Can you work these out from the model? Positions are in its coordinate system, mm. A direction names the side the tool comes from. Coordinates: 2 decimals unless noted, no trailing zeros. Order: outer loops, then holes, each group sorted by start corner. A loop starts at its lowest first (then second) coordinate and runs counter-clockwise, first axis right, second up. Notation, with made-up numbers: (23, 10.25) - (69, 10.25) arc R23 ccw to (69, 31.25) - close; hole circle Ø3 at (58.5, -34). An arc over 180 degrees is marked (long way). Return JSON: item names as keys, results as strings. Group by question number.
1) Imagine slicing it at A-A (z = 50). Write out the boundary of the cut face in (x, y).
2) Which directions (+Z, -Z, +X, -X, +Y, -Y) give clear straight access to the entire face, cutting with the end or side of a thin tool? Please do faces 1 (the face through (-1, 35, 120)), 2 (the face through (43, 5, 54)).
3) If I drill on line 1 along Z through (x, y) = (-91, 3); line 2 along X through (y, z) = (6, -111); line 3 along X through (y, z) = (4, -50), over which ranges is the centre line in solid material (lowest first)?
4) Imagine slicing it at C-C (y = 46.5). Write out the boundary of the cut face in (x, z).
5) Imagine slicing it at B-B (x = -40). Write out the boundary of the cut face in (y, z), and give its area (3 significant figures).
6) For pin 1 Ø1.5 at (x, z) = (68.5, 76.5) entering from +Y; pin 2 Ø8 at (x, z) = (40, 50) entering from -Y, each with a flat end and sliding along its axis, tell me the tip position at first contact or that it passes through.
7) Imagine slicing it at D-D (x = 54.5). Write out the boundary of the cut face in (y, z).
8) If we mould it in two halves opening along X, with no side actions, what happens to faces 3 (the face through (-103, 30, 2)), 4 (the face through (103, 30, 2)), 5 (the face through (100, 35, 2))? For each: pulls with the +X half, pulls with the -X half, needs draft (parallel to the pull), parting line crosses it, or undercut.
```python
from build123d import *

# Parameters (mm, degrees)
SKETCH1_W           = 206
SKETCH1_H           = 246
BOSS_EXTRUDE1_DEPTH = 60
SKETCH2_W           = 200
SKETCH2_H           = 240
CUT_EXTRUDE1_DEPTH  = 50
CUT_EXTRUDE3_DEPTH  = 172.283390905
SKETCH4_R           = 5
CUT_EXTRUDE4_DEPTH  = 10


with BuildPart() as part:
    # Sketch1 → Boss-Extrude1 (new body)
    with BuildSketch(Plane(origin=(0, 0, 0), x_dir=(1, 0, 0), z_dir=(0, 1, 0))):
        Rectangle(SKETCH1_W, SKETCH1_H)
    extrude(amount=BOSS_EXTRUDE1_DEPTH)

    # Sketch2 → Cut-Extrude1 (cut)
    with BuildSketch(Plane(origin=(0, 60, 0), x_dir=(1, 0, 0), z_dir=(0, 1, 0))):
        Rectangle(SKETCH2_W, SKETCH2_H)
    extrude(amount=-CUT_EXTRUDE1_DEPTH, mode=Mode.SUBTRACT)

    # Sketch3 → Cut-Extrude3 (cut, through all)
    with BuildSketch(Plane.XZ):
        with BuildLine():
            Line((-91, 106), (-91, 111))
            Line((-91, 111), (-86, 111))
            ThreePointArc((-86, 111), (-94.535533906, 114.535533906), (-91, 106))
        make_face()
        with BuildLine():
            Line((-86, 111), (-91, 111))
            Line((-91, 111), (-91, 106))
            ThreePointArc((-91, 106), (-87.464466094, 107.464466094), (-86, 111))
        make_face()
        with BuildLine():
            ThreePointArc((96, 111), (91, 116), (86, 111))
            Line((86, 111), (91, 111))
            Line((91, 111), (91, 106))
            ThreePointArc((91, 106), (94.535533906, 107.464466094), (96, 111))
        make_face()
        with BuildLine():
            Line((91, 111), (86, 111))
            ThreePointArc((86, 111), (87.464466094, 107.464466094), (91, 106))
            Line((91, 106), (91, 111))
        make_face()
        with BuildLine():
            ThreePointArc((96, -111), (94.535533906, -107.464466094), (91, -106))
            Line((91, -106), (91, -111))
            Line((91, -111), (86, -111))
            ThreePointArc((86, -111), (91, -116), (96, -111))
        make_face()
        with BuildLine():
            Line((91, -111), (91, -106))
            ThreePointArc((91, -106), (87.464466094, -107.464466094), (86, -111))
            Line((86, -111), (91, -111))
        make_face()
        with BuildLine():
            ThreePointArc((-86, -111), (-87.464466094, -107.464466094), (-91, -106))
            Line((-91, -106), (-91, -111))
            Line((-91, -111), (-86, -111))
        make_face()
        with BuildLine():
            Line((-91, -111), (-91, -106))
            ThreePointArc((-91, -106), (-94.535533906, -114.535533906), (-86, -111))
            Line((-86, -111), (-91, -111))
        make_face()
    extrude(amount=-CUT_EXTRUDE3_DEPTH, mode=Mode.SUBTRACT)

    # Sketch4 → Cut-Extrude4 (cut)
    with BuildSketch(Plane.XZ):
        with Locations(Location((40, -50, 0), (0, 0, 270))):
            Circle(SKETCH4_R)
        with Locations(Location((-40, -50, 0), (0, 0, 270))):
            Circle(SKETCH4_R)
        with Locations(Location((-40, 50, 0), (0, 0, 270))):
            Circle(SKETCH4_R)
        with Locations(Location((40, 50, 0), (0, 0, 270))):
            Circle(SKETCH4_R)
    extrude(amount=-CUT_EXTRUDE4_DEPTH, mode=Mode.SUBTRACT)


solid = part.part
```
Calculated:
{
 "1": {"outline": "(-103, 0) - (-45, 0) - (-45, 10) - (-100, 10) - (-100, 60) - (-103, 60) - close; (-35, 0) - (35, 0) - (35, 10) - (-35, 10) - close; (45, 0) - (103, 0) - (103, 60) - (100, 60) - (100, 10) - (45, 10) - close"},
 "2": {"face 1": "+Y", "face 2": "+Y, -Y"},
 "3": {"line 1": "-123 to -116, -106 to 106, 116 to 123", "line 2": "-103 to -96, -86 to 86, 96 to 103", "line 3": "-103 to -45, -35 to 35, 45 to 103"},
 "4": {"outline": "(-103, -123) - (103, -123) - (103, 123) - (-103, 123) - close; hole (-100, -120) - (100, -120) - (100, 120) - (-100, 120) - close"},
 "5": {"outline": "(0, -123) - (60, -123) - (60, -120) - (10, -120) - (10, -55) - (0, -55) - close; (0, -45) - (10, -45) - (10, 45) - (0, 45) - close; (0, 55) - (10, 55) - (10, 120) - (60, 120) - (60, 123) - (0, 123) - close", "area": "2,560 mm2"},
 "6": {"pin 1": "y = 10", "pin 2": "through"},
 "7": {"outline": "(0, -123) - (60, -123) - (60, -120) - (10, -120) - (10, 120) - (60, 120) - (60, 123) - (0, 123) - close"},
 "8": {"face 3": "pulls with the -X half", "face 4": "pulls with the +X half", "face 5": "undercut"}
}
